```python
from build123d import *

# Parameters (mm, degrees)
F0_W        = 257
F0_H        = 70
F1_DEPTH    = 19
F2_W        = 3
F2_H        = 3
F3_DEPTH    = 257.001
F4_W        = 6
F4_H        = 17
F5_DEPTH    = 257.001
F6_T1_DEPTH = 159.7239535427


# Not quite as in the source:
# - a fillet or chamfer that OpenCascade refuses, or shapes differently, is made with other operations: its cross-section is extruded or revolved along the edge and cut away or added


with BuildPart() as f1:
    # F0 (on Right) → F1 (new body)
    with BuildSketch(Plane.YZ):
        with Locations((-128.5, 35)):
            Rectangle(F0_W, F0_H)
    extrude(amount=F1_DEPTH)

    # F2 (on face) → F3 (cut, through all)
    with BuildSketch(Plane.XZ.offset(257)):
        with Locations((1.5, 6.5)):
            Rectangle(F2_W, F2_H)
    extrude(amount=-F3_DEPTH, mode=Mode.SUBTRACT)

    # F4 (on face) → F5 (cut, through all)
    with BuildSketch(Plane.XZ.offset(257)):
        with Locations((16, 18.5)):
            Rectangle(F4_W, F4_H)
    extrude(amount=-F5_DEPTH, mode=Mode.SUBTRACT)

    # F6: chamfer of 19 on 1 edges, made by hand

    # F6_s2 → F6_t1 (cut)
    with BuildSketch(Plane.XY.offset(-40.8619767714)):
        Polygon((19, 0), (0, -19), (0, 0), align=None)
    extrude(amount=F6_T1_DEPTH, mode=Mode.SUBTRACT)


solid = f1.part
```
The listing builds one solid part. Answer for the finished solid, in the listing's coordinates (mm). A direction names the side the tool comes from. Coordinates: 2 decimals unless noted, no trailing zeros. Loops run counter-clockwise (first coordinate to the right, second up) from the corner with the lowest first, then second, coordinate; pieces in that order, holes last. Notation, with made-up numbers: (-9, -32.75) - (27, -32.75) arc R17 cw to (27, -6.75) - close; hole circle Ø2 at (67.25, -35). An arc over 180 degrees is marked (long way). Write item = value, one per line.
1) Find the intervals of material crossed by line 1 along Z through (x, y) = (1.75, -225.5); line 2 along Z through (x, y) = (16, -158.5); line 3 along X through (y, z) = (-64, 26), in increasing order.
Responses:
line_1 = 0 to 5, 8 to 70
line_2 = 0 to 10, 27 to 70
line_3 = 0 to 13
2) Each of these flat-tipped pins is pushed along its axis until it touches: P1, Ø0.9, axis at y = -83, z = 7, coming from the -X side; P2, Ø8.5, axis at y = -106.5, z = 16, coming from the +X side; P3, Ø2, axis at x = 3, z = 59, coming from the +Y side. Where does it stop, or does it pass through?
Responses:
P1 = 3
P2 = 13
P3 = -15
3) Section C-C (z = 17) is taken. Determine the outline of the cut face in (x, y).
Responses:
outline = (0, -257) - (13, -257) - (13, -6) - (0, -19) - close
4) Section D-D (z = 61.5) is taken. Determine the outline of the cut face in (x, y).
Responses:
outline = (0, -257) - (19, -257) - (19, 0) - (0, -19) - close
5) Section B-B (y = -53) is taken. Determine the outline of the cut face in (x, z), plus the area to 3 significant figures.
Responses:
outline = (0, 0) - (19, 0) - (19, 10) - (13, 10) - (13, 27) - (19, 27) - (19, 70) - (0, 70) - (0, 8) - (3, 8) - (3, 5) - (0, 5) - close
area = 1,220 mm^2
6) Section A-A (x = 15.25) is taken. Determine the outline of the cut face in (y, z), plus the area to 3 significant figures.
Responses:
outline = (-257, 0) - (-3.75, 0) - (-3.75, 10) - (-257, 10) - close; (-257, 27) - (-3.75, 27) - (-3.75, 70) - (-257, 70) - close
area = 13,400 mm^2
7) Which of the six approach directions +Z, -Z, +X, -X, +Y, -Y give full straight-line access (tool end or side, diameter ignored) to faces 1 (the face through (0, -140, 39)), 2 (the face through (16, -130, 10))?
Responses:
face_1 = +Z, -Z, -X, +Y, -Y
face_2 = +X, +Y, -Y
